```python
from build123d import *

# Parameters (mm, degrees)
SKETCH1_W           = 307.7
SKETCH1_H           = 250
BOSS_EXTRUDE1_DEPTH = 6.35
SKETCH2_R           = 4
SKETCH2_W           = 6.35
SKETCH2_H           = 50
CUT_EXTRUDE1_DEPTH  = 397.509284254


with BuildPart() as part:
    # Sketch1 → Boss-Extrude1 (new body)
    with BuildSketch(Plane.XY):
        with Locations((153.85, 125)):
            Rectangle(SKETCH1_W, SKETCH1_H)
    extrude(amount=BOSS_EXTRUDE1_DEPTH)

    # Sketch2 → Cut-Extrude1 (cut, through all)
    with BuildSketch(Plane.XY.offset(6.35)):
        with Locations((290.35, 237.3)):
            Circle(SKETCH2_R)
        with Locations((304.525, 75)):
            Rectangle(SKETCH2_W, SKETCH2_H)
        with Locations((304.525, 185)):
            Rectangle(SKETCH2_W, SKETCH2_H)
        with Locations((3.175, 75)):
            Rectangle(SKETCH2_W, SKETCH2_H)
        with Locations((3.175, 185)):
            Rectangle(SKETCH2_W, SKETCH2_H)
    extrude(amount=-CUT_EXTRUDE1_DEPTH, mode=Mode.SUBTRACT)


solid = part.part
```
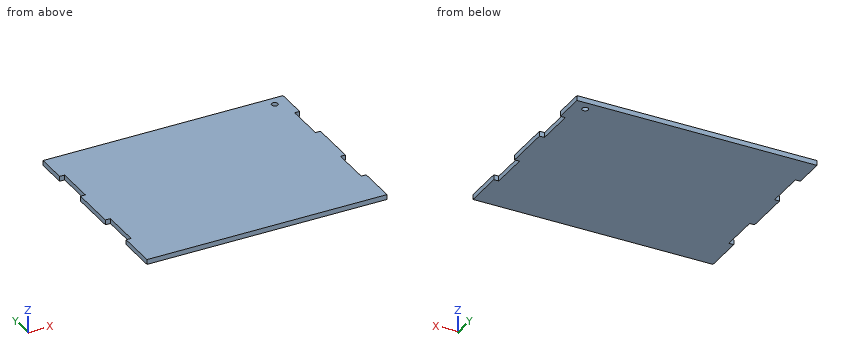
Part model, mm, in its own coordinate system. Coordinates: 2 decimals unless noted, no trailing zeros. Loops run counter-clockwise (first coordinate to the right, second up) from the corner with the lowest first, then second, coordinate; pieces in that order, holes last. Notation, with made-up numbers: (86, 8) - (102, 8) arc R25 ccw to (102, 26) - close; hole circle Ø1 at (-20, 14). An arc over 180 degrees is marked (long way). Write item = value, one per line. Start each with the question number.
Item 1: Flat gauge pins, fed straight in: pin 1 Ø3 at (x, z) = (3.5, 3) entering from -Y; pin 2 Ø3 at (y, z) = (186.5, 4) entering from +X; pin 3 Ø1.9 at (y, z) = (176.5, 4) entering from -X. Where does each tip first touch, or does it go through?
Item 2: Cut at C-C, the plane z = 1.5. Give the cut face in (x, y).
Item 3: Cut at B-B, the plane y = 237.3. Give the cut face in (x, z).
Item 4: Cut at A-A, the plane x = 290.35. Give the cut face in (y, z).
Item 5: Cut at D-D, the plane y = 189. Give the cut face in (x, z).
Item 6: Wall check: L1, parallel to Y at x = 290.35, z = 4.5; L2, parallel to X at y = 166, z = 3. Give the ranges that are in metal, low to high. Write a range as from..to.
The answers:
q1.pin_1 = 0
q1.pin_2 = 301.35
q1.pin_3 = 6.35
q2.outline = (0, 0) - (307.7, 0) - (307.7, 50) - (301.35, 50) - (301.35, 100) - (307.7, 100) - (307.7, 160) - (301.35, 160) - (301.35, 210) - (307.7, 210) - (307.7, 250) - (0, 250) - (0, 210) - (6.35, 210) - (6.35, 160) - (0, 160) - (0, 100) - (6.35, 100) - (6.35, 50) - (0, 50) - close; hole circle Ø8 at (290.35, 237.3)
q3.outline = (0, 0) - (286.35, 0) - (286.35, 6.35) - (0, 6.35) - close; (294.35, 0) - (307.7, 0) - (307.7, 6.35) - (294.35, 6.35) - close
q4.outline = (0, 0) - (233.3, 0) - (233.3, 6.35) - (0, 6.35) - close; (241.3, 0) - (250, 0) - (250, 6.35) - (241.3, 6.35) - close
q5.outline = (6.35, 0) - (301.35, 0) - (301.35, 6.35) - (6.35, 6.35) - close
q6.L1 = 0..233.3, 241.3..250
q6.L2 = 6.35..301.35
